from build123d import *

# Parameters (mm, degrees)
SZKIC1_W                    = 95
SZKIC1_H                    = 18
DODANIE_WYCI_GNI_CIE1_DEPTH = 1.6
GNIAZDO1_START              = -34.197888829
GNIAZDO1_OUTLINE_W          = 4.7
GNIAZDO1_OUTLINE_H          = 1.6
GNIAZDO1_DEPTH              = 1.6
GNIAZDO1_START_2            = -17.697888829
GNIAZDO1_2_OUTLINE_W        = 4.7
GNIAZDO1_2_OUTLINE_H        = 1.6
GNIAZDO1_2_DEPTH            = 1.6
GNIAZDO1_START_3            = -1.197888829
GNIAZDO1_3_OUTLINE_W        = 4.7
GNIAZDO1_3_OUTLINE_H        = 1.6
GNIAZDO1_3_DEPTH            = 1.6
GNIAZDO1_START_4            = 15.302111171
GNIAZDO1_4_OUTLINE_W        = 4.7
GNIAZDO1_4_OUTLINE_H        = 1.6
GNIAZDO1_4_DEPTH            = 1.6
GNIAZDO1_START_5            = 31.802111171
GNIAZDO1_5_OUTLINE_W        = 4.7
GNIAZDO1_5_OUTLINE_H        = 1.6
GNIAZDO1_5_DEPTH            = 1.6
WYTNIJ_WYCI_GNI_CIE2_DEPTH  = 1.6
ZAOKR_GLENIE1_R             = 3.5
SZKIC37_R                   = 1.5
WYTNIJ_WYCI_GNI_CIE3_DEPTH  = 1.6
SZKIC38_R                   = 1.5
WYTNIJ_WYCI_GNI_CIE4_DEPTH  = 60.867696542
SZKIC39_R                   = 0.375000457
SZKIC39_R_2                 = 0.375246396
SZKIC39_R_3                 = 0.375
SZKIC39_R_4                 = 0.375428794
SZKIC39_R_5                 = 0.37501816
SZKIC39_R_6                 = 0.375001619
SZKIC39_R_7                 = 0.375794755
WYTNIJ_WYCI_GNI_CIE5_DEPTH  = 1.6


# Read off the part's stored shape, not the designer's step: Gniazdo1
with BuildPart() as part:
    # Szkic1 → Dodanie-wyciągnięcie1 (new body)
    with BuildSketch(Plane.XY):
        with Locations((-1.797888829, 24.930800849)):
            Rectangle(SZKIC1_W, SZKIC1_H)
    extrude(amount=DODANIE_WYCI_GNI_CIE1_DEPTH)

    # Gniazdo1 outline → Gniazdo1 (cut)
    with BuildSketch(Plane.YZ.offset(GNIAZDO1_START)):
        with Locations((27.580800849, 0.8)):
            Rectangle(GNIAZDO1_OUTLINE_W, GNIAZDO1_OUTLINE_H)
    extrude(amount=GNIAZDO1_DEPTH, mode=Mode.SUBTRACT)

    # Gniazdo1 2 outline → Gniazdo1 2 (cut)
    with BuildSketch(Plane.YZ.offset(GNIAZDO1_START_2)):
        with Locations((27.580800849, 0.8)):
            Rectangle(GNIAZDO1_2_OUTLINE_W, GNIAZDO1_2_OUTLINE_H)
    extrude(amount=GNIAZDO1_2_DEPTH, mode=Mode.SUBTRACT)

    # Gniazdo1 3 outline → Gniazdo1 3 (cut)
    with BuildSketch(Plane.YZ.offset(GNIAZDO1_START_3)):
        with Locations((27.580800849, 0.8)):
            Rectangle(GNIAZDO1_3_OUTLINE_W, GNIAZDO1_3_OUTLINE_H)
    extrude(amount=GNIAZDO1_3_DEPTH, mode=Mode.SUBTRACT)

    # Gniazdo1 4 outline → Gniazdo1 4 (cut)
    with BuildSketch(Plane.YZ.offset(GNIAZDO1_START_4)):
        with Locations((27.580800849, 0.8)):
            Rectangle(GNIAZDO1_4_OUTLINE_W, GNIAZDO1_4_OUTLINE_H)
    extrude(amount=GNIAZDO1_4_DEPTH, mode=Mode.SUBTRACT)

    # Gniazdo1 5 outline → Gniazdo1 5 (cut)
    with BuildSketch(Plane.YZ.offset(GNIAZDO1_START_5)):
        with Locations((27.580800849, 0.8)):
            Rectangle(GNIAZDO1_5_OUTLINE_W, GNIAZDO1_5_OUTLINE_H)
    extrude(amount=GNIAZDO1_5_DEPTH, mode=Mode.SUBTRACT)

    # Szkic35 → Wytnij-wyciągnięcie2 (cut)
    with BuildSketch(Plane.XY.offset(1.6)):
        Polygon((-34.297888829, 30.030800849), (-34.297888829, 25.130800849), (-32.597888829, 25.130800849), (-32.597888829, 30.030800849), (-34.197888829, 30.030800849), align=None)
        Polygon((-17.797888829, 30.030800849), (-17.797888829, 25.130800849), (-16.097888829, 25.130800849), (-16.097888829, 30.030800849), (-17.697888829, 30.030800849), align=None)
        Polygon((-1.297888829, 30.030800849), (-1.297888829, 25.130800849), (0.402111171, 25.130800849), (0.402111171, 30.030800849), (-1.197888829, 30.030800849), align=None)
        Polygon((15.202111171, 30.030800849), (15.202111171, 25.130800849), (16.902111171, 25.130800849), (16.902111171, 30.030800849), (15.302111171, 30.030800849), align=None)
        Polygon((31.702111171, 30.030800849), (31.702111171, 25.130800849), (33.402111171, 25.130800849), (33.402111171, 30.030800849), (31.802111171, 30.030800849), align=None)
    extrude(amount=-WYTNIJ_WYCI_GNI_CIE2_DEPTH, mode=Mode.SUBTRACT)

    # Zaokrąglenie1
    zaokr_glenie1_edges = [part.edges().sort_by_distance(p)[0] for p in [
        (45.702111171, 33.930800849, 0.8),
    ]]
    fillet(zaokr_glenie1_edges, radius=ZAOKR_GLENIE1_R)

    # Szkic37 → Wytnij-wyciągnięcie3 (cut)
    with BuildSketch(Plane.XY.offset(1.6)):
        with Locations((39.502111171, 24.930800849)):
            Circle(SZKIC37_R)
        with Locations((-43.097888829, 24.930800849)):
            Circle(SZKIC37_R)
    extrude(amount=-WYTNIJ_WYCI_GNI_CIE3_DEPTH, mode=Mode.SUBTRACT)

    # Szkic38 → Wytnij-wyciągnięcie4 (cut, through all)
    with BuildSketch(Plane.XY.offset(1.6)):
        with Locations((-9.297888829, 24.930800849)):
            Circle(SZKIC38_R)
    extrude(amount=-WYTNIJ_WYCI_GNI_CIE4_DEPTH, mode=Mode.SUBTRACT)

    # Szkic39 → Wytnij-wyciągnięcie5 (cut)
    with BuildSketch(Plane.XY.offset(1.6)):
        with Locations((-34.298474307, 25.505800849)):
            Circle(SZKIC39_R)
        with Locations((-32.611485055, 25.505800849)):
            Circle(SZKIC39_R_2)
        with Locations((-17.797888829, 25.505800849)):
            Circle(SZKIC39_R_3)
        with Locations((-16.079950616, 25.505800849)):
            Circle(SZKIC39_R_4)
        with Locations((-1.301579386, 25.505800849)):
            Circle(SZKIC39_R_5)
        with Locations((0.402111171, 25.505800849)):
            Circle(SZKIC39_R_3)
        with Locations((15.203212962, 25.505800849)):
            Circle(SZKIC39_R_6)
        with Locations((16.902111171, 25.505800849)):
            Circle(SZKIC39_R_3)
        with Locations((31.702111171, 25.505800849)):
            Circle(SZKIC39_R_3)
        with Locations((33.377683776, 25.505800849)):
            Circle(SZKIC39_R_7)
        with Locations((-34.297888829, 29.655800849)):
            Circle(SZKIC39_R_3)
        with Locations((-32.597888829, 29.655800849)):
            Circle(SZKIC39_R_3)
        with Locations((-17.797888829, 29.655800849)):
            Circle(SZKIC39_R_3)
        with Locations((-16.097888829, 29.655800849)):
            Circle(SZKIC39_R_3)
        with Locations((-1.297888829, 29.655800849)):
            Circle(SZKIC39_R_3)
        with Locations((0.402111171, 29.655800849)):
            Circle(SZKIC39_R_3)
        with Locations((15.203212962, 29.655800849)):
            Circle(SZKIC39_R_6)
        with Locations((16.902111171, 29.655800849)):
            Circle(SZKIC39_R_3)
        with Locations((31.702111171, 29.655800849)):
            Circle(SZKIC39_R_3)
        with Locations((33.377683776, 29.655800849)):
            Circle(SZKIC39_R_7)
    extrude(amount=-WYTNIJ_WYCI_GNI_CIE5_DEPTH, mode=Mode.SUBTRACT)


solid = part.part
CAD build for the part. Positions are in the model's coordinates, mm. A direction names the side the tool comes from. Coordinates: 2 decimals unless noted, no trailing zeros. Write item = value, one per line. Start each with the question number.
Q1. Drill centre lines: L1, parallel to X at y = 28, z = 0.35; L2, parallel to Y at x = 17, z = 1; L3, parallel to Y at x = 32.5, z = 0.4. Where is each one in solid material? Low to high.
Q2. Which spindle directions (+Z, -Z, +X, -X, +Y, -Y) get a long thin tool onto all of the face, cutting with end or side? Do faces 1 (the flat face through (-17.798, 28, 1)), 2 (the flat face through (-2, 25, 0)). Say none if no direction does.
Q3. Flat gauge pin, fed straight in: pin 1 Ø10 at (x, y) = (17.5, 28.5) entering from -Z. Where does the tip first touch, or does it go through?
Q4. Pull direction X, two halves, no side cores. Call faces 3 (the cylindrical face through (-7.867, 25.381, 0.811)), 4 (the flat face through (-49.298, 25, 1)), 5 (the cylindrical face through (44.7, 32.88, 0.81)): pulls with the +X half, pulls with the -X half, needs draft (parallel to the pull), parting line crosses it, or undercut.
Q5. Cut at A-A, the plane z = 1.25. Give the number of separate pieces and of enclosed holes in the cut face, then the cut area to 3 significant figures.
Computed:
q1.L1 = -49.3 to -34.3, -32.6 to -17.8, -16.1 to -1.3, 0.4 to 15.2, 16.9 to 31.7, 33.4 to 45.7
q1.L2 = 15.93 to 25.14, 25.87 to 29.29, 30.02 to 33.93
q1.L3 = 15.93 to 25.13, 30.03 to 33.93
q2.face_1 = +Z, -Z
q2.face_2 = -Z, +X, -X, +Y, -Y
q3.pin_1 = 0
q4.face_3 = undercut
q4.face_4 = pulls with the -X half
q4.face_5 = pulls with the +X half
q5.separate_pieces = 1
q5.enclosed_holes = 8
q5.area = 1,640 mm²
